Source: CAD feature listing. Evaluate the final solid. Frame: model axes, mm. Coordinates: 2 decimals unless noted, no trailing zeros. Order: outer loops, then holes, each group sorted by start corner. A loop starts at its lowest first (then second) coordinate and runs counter-clockwise, first axis right, second up. Notation, with made-up numbers: (76, -36.75) - (119, -36.75) arc R18 cw to (119, -4.75) - close; hole circle Ø5 at (68, -27.75). An arc over 180 degrees is marked (long way). One line per question, with ' | ' between items. Start each with the question number.
(1) Section D-D (y = 3.81). Return the cut outline in (x, z).
(2) Section B-B (z = 7). Return the cut outline in (x, y), then the cut area to 3 significant figures.
(3) Contact query for flat-ended pins moving along their axis: P1, Ø4, axis at x = 24.5, y = 48.5, coming from the +Z side; P2, Ø3.5, axis at y = 5, z = 4.5, coming from the -X side; P3, Ø3, axis at x = 3.81, y = 3.81, coming from the -Z side; P4, Ø3.5, axis at y = 4, z = 4.5, coming from the +X side. Output: stop coordinate, or through.
(4) Line query: line 1 along X through (y, z) = (7.5, 4); line 2 along Y through (x, z) = (3.81, 0.55); line 3 along Z through (x, y) = (39.5, 21). Output: solid intervals per line, ascending.
(5) Section A-A (y = 57.15). Return the cut outline in (x, z), then the cut area to 3 significant figures.
(6) Section C-C (x = 3.81). Return the cut outline in (y, z).
from build123d import *

# Parameters (mm, degrees)
SKETCH1_W           = 100.076
SKETCH1_H           = 60.96
SKETCH1_R           = 1.5875
BOSS_EXTRUDE1_DEPTH = 1.5748
SKETCH2_W           = 10.795
SKETCH2_H           = 7.62
SKETCH2_W_2         = 12.7
BOSS_EXTRUDE2_DEPTH = 7.112


with BuildPart() as part:
    # Sketch1 → Boss-Extrude1 (new body)
    with BuildSketch(Plane.XY):
        with Locations((50.038, 30.48)):
            Rectangle(SKETCH1_W, SKETCH1_H)
        with Locations((3.81, 57.15)):
            Circle(SKETCH1_R, mode=Mode.SUBTRACT)
        with Locations((96.266, 57.15)):
            Circle(SKETCH1_R, mode=Mode.SUBTRACT)
        with Locations((96.266, 3.81)):
            Circle(SKETCH1_R, mode=Mode.SUBTRACT)
        with Locations((3.81, 3.81)):
            Circle(SKETCH1_R, mode=Mode.SUBTRACT)
    extrude(amount=BOSS_EXTRUDE1_DEPTH)

    # Sketch2 → Boss-Extrude2 (add)
    with BuildSketch(Plane.XY.offset(1.5748)):
        with Locations((12.446, 3.81)):
            Rectangle(SKETCH2_W, SKETCH2_H)
        with Locations((85.344, 3.81)):
            Rectangle(SKETCH2_W_2, SKETCH2_H)
    extrude(amount=BOSS_EXTRUDE2_DEPTH)


solid = part.part
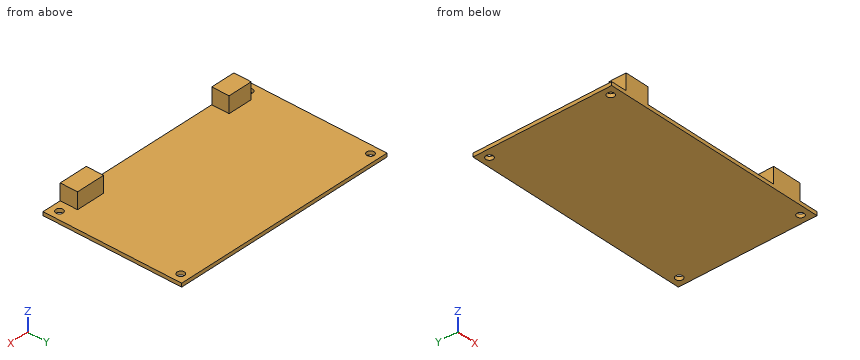
Response values:
1) outline: (0, 0) - (2.22, 0) - (2.22, 1.57) - (0, 1.57) - close; (5.4, 0) - (94.68, 0) - (94.68, 1.57) - (91.69, 1.57) - (91.69, 8.69) - (78.99, 8.69) - (78.99, 1.57) - (17.84, 1.57) - (17.84, 8.69) - (7.05, 8.69) - (7.05, 1.57) - (5.4, 1.57) - close; (97.85, 0) - (100.08, 0) - (100.08, 1.57) - (97.85, 1.57) - close
2) outline: (7.05, 0) - (17.84, 0) - (17.84, 7.62) - (7.05, 7.62) - close; (78.99, 0) - (91.69, 0) - (91.69, 7.62) - (78.99, 7.62) - close | area: 179 mm²
3) P1: stops at z = 1.57 | P2: stops at x = 7.05 | P3: passes through | P4: stops at x = 91.69
4) line 1: x = 7.05 to 17.84, 78.99 to 91.69 | line 2: y = 0 to 2.22, 5.4 to 55.56, 58.74 to 60.96 | line 3: z = 0 to 1.57
5) outline: (0, 0) - (2.22, 0) - (2.22, 1.57) - (0, 1.57) - close; (5.4, 0) - (94.68, 0) - (94.68, 1.57) - (5.4, 1.57) - close; (97.85, 0) - (100.08, 0) - (100.08, 1.57) - (97.85, 1.57) - close | area: 148 mm²
6) outline: (0, 0) - (2.22, 0) - (2.22, 1.57) - (0, 1.57) - close; (5.4, 0) - (55.56, 0) - (55.56, 1.57) - (5.4, 1.57) - close; (58.74, 0) - (60.96, 0) - (60.96, 1.57) - (58.74, 1.57) - close
